The model under review builds one solid part; all positions refer to its coordinate system, in mm. A direction names the side the tool comes from. Round coordinates to 2 decimals unless told otherwise and drop trailing zeros. Write each loop counter-clockwise with the first axis right and the second up, starting at its lowest first coordinate (ties: lowest second). Pieces come first, ordered by that corner, then holes. Notation, with made-up numbers: (22.5, -7) -> (76.5, -7) arc R19 ccw to (76.5, 3) -> close; hole circle Ø5 at (34.5, 16.25). An arc over 180 degrees is marked (long way). Use CSV: the item, a comma, the result in double quotes. Start each with the question number.
1) Machinability: for faces 4 (the face through (-77, 7, -30)), 5 (the face through (-77, 15, -9.2)), 6 (the face through (-77, 20.8, -15)), 7 (the face through (-77, 15, -20.8)), which of the approach directions +Z, -Z, +X, -X, +Y, -Y give a long, thin tool a straight path to every point of the face, cutting with its end or side? Answer none if there is none.
2) Take a section at A-A, the plane z = -15. Give the boundary of the cut face in (x, y).
3) Mouldability with a two-part tool opening along Z and no side actions: class faces 1 (the face through (-77, 0, -7)), 2 (the face through (-77, 9.2, -15)), 3 (the face through (-77, 23, 0)) as released by +Z, released by -Z, zero draft, split by the parting line, or undercut.
4) Take a section at B-B, the plane y = 15. Give the boundary of the cut face in (x, z).
5) For pin 1 Ø6 at (y, z) = (25.5, -12) entering from +X; pin 2 Ø1.9 at (x, z) = (-127, -29) entering from -Y; pin 3 Ø3.5 at (x, y) = (0.5, 15) entering from +Z; pin 4 Ø1 at (x, y) = (-47, 14) entering from -Z, all flat-tipped, find the tip position at first contact; note any pin that passes through.
6) Wall thickness on probe 1 along Z at (x, y) = (9.5, 25); probe 2 along Z at (x, y) = (-36, 15); probe 3 along Y at (x, z) = (-83.5, -8): over which ranges is each line inside the solid? List them lowest first. Write a range as [from, to].
from build123d import *
from build123d.topology import SkipClean

# Parameters (mm, degrees)
SKETCH1_R           = 3.4
BOSS_EXTRUDE2_DEPTH = 100
FILLET5_R           = 2.5
FILLET6_R           = 1.5
FILLET7_R           = 1.5
FILLET8_R           = 1
SKETCH3_R           = 3.4
BOSS_EXTRUDE3_DEPTH = 140
SKETCH7_R           = 3.4
BOSS_EXTRUDE4_DEPTH = 120


with BuildPart() as part:
    # Sketch1 → Boss-Extrude2 (new body)
    with BuildSketch(Plane(origin=(0, 0, 0), x_dir=(0, 0, -1), z_dir=(1, 0, 0))):
        Polygon((10.9, 0), (10.9, 2.4), (6.75, 2.4), (6.75, 5.05), (10.9, 9.2), (19.1, 9.2), (23.25, 5.05), (23.25, 2.4), (19.1, 2.4), (19.1, 0), (30, 0), (30, 10.9), (27.6, 10.9), (27.6, 6.75), (24.95, 6.75), (20.8, 10.9), (20.8, 19.1), (24.95, 23.25), (27.6, 23.25), (27.6, 19.1), (30, 19.1), (30, 30), (19.1, 30), (19.1, 27.6), (23.25, 27.6), (23.25, 24.95), (19.1, 20.8), (10.9, 20.8), (6.75, 24.95), (6.75, 27.6), (10.9, 27.6), (10.9, 30), (0, 30), (0, 19.1), (2.4, 19.1), (2.4, 23.25), (5.05, 23.25), (9.2, 19.1), (9.2, 10.9), (5.05, 6.75), (2.4, 6.75), (2.4, 10.9), (0, 10.9), (0, 0), align=None)
        with Locations((15, 15)):
            Circle(SKETCH1_R, mode=Mode.SUBTRACT)
    extrude(amount=BOSS_EXTRUDE2_DEPTH)

    # Fillet5
    fillet5_edges = [part.edges().sort_by_distance(p)[0] for p in [
        (50, 30, 0),
        (50, 30, -30),
        (50, 0, -30),
        (50, 0, 0),
    ]]
    fillet(fillet5_edges, radius=FILLET5_R)

    # Fillet6
    fillet6_edges = [part.edges().sort_by_distance(p)[0] for p in [
        (50, 10.9, -9.2),
        (50, 19.1, -9.2),
        (50, 19.1, -20.8),
        (50, 10.9, -20.8),
        (50, 9.2, -19.1),
        (50, 9.2, -10.9),
    ]]
    fillet(fillet6_edges, radius=FILLET6_R)

    # Fillet7
    fillet7_edges = [part.edges().sort_by_distance(p)[0] for p in [
        (50, 20.8, -10.9),
        (50, 20.8, -19.1),
    ]]
    fillet(fillet7_edges, radius=FILLET7_R)

    # Fillet8
    fillet8_edges = [part.edges().sort_by_distance(p)[0] for p in [
        (50, 6.75, -2.4),
        (50, 23.25, -2.4),
        (50, 27.6, -6.75),
        (50, 27.6, -23.25),
        (50, 23.25, -27.6),
        (50, 6.75, -27.6),
        (50, 2.4, -23.25),
        (50, 2.4, -6.75),
    ]]
    fillet(fillet8_edges, radius=FILLET8_R)

    # Sketch3 → Boss-Extrude3 (add)
    with BuildSketch(Plane(origin=(0, 0, 0), x_dir=(0, 0, -1), z_dir=(1, 0, 0))):
        with BuildLine():
            Line((10.9, 27.6), (10.9, 30))
            Line((10.9, 30), (2.5, 30))
            ThreePointArc((2.5, 30), (0.732233047, 29.267766953), (0, 27.5))
            Line((0, 27.5), (0, 19.1))
            Line((0, 19.1), (2.4, 19.1))
            Line((2.4, 19.1), (2.4, 22.25))
            ThreePointArc((2.4, 22.25), (2.692893219, 22.957106781), (3.4, 23.25))
            Line((3.4, 23.25), (5.05, 23.25))
            Line((5.05, 23.25), (8.760660172, 19.539339828))
            ThreePointArc((8.760660172, 19.539339828), (9.085819299, 19.052704805), (9.2, 18.478679656))
            Line((9.2, 18.478679656), (9.2, 11.521320344))
            ThreePointArc((9.2, 11.521320344), (9.085819299, 10.947295195), (8.760660172, 10.460660172))
            Line((8.760660172, 10.460660172), (5.05, 6.75))
            Line((5.05, 6.75), (3.4, 6.75))
            ThreePointArc((3.4, 6.75), (2.692893219, 7.042893219), (2.4, 7.75))
            Line((2.4, 7.75), (2.4, 10.9))
            Line((2.4, 10.9), (0, 10.9))
            Line((0, 10.9), (0, 2.5))
            ThreePointArc((0, 2.5), (0.732233047, 0.732233047), (2.5, 0))
            Line((2.5, 0), (10.9, 0))
            Line((10.9, 0), (10.9, 2.4))
            Line((10.9, 2.4), (7.75, 2.4))
            ThreePointArc((7.75, 2.4), (7.042893219, 2.692893219), (6.75, 3.4))
            Line((6.75, 3.4), (6.75, 5.05))
            Line((6.75, 5.05), (10.460660172, 8.760660172))
            ThreePointArc((10.460660172, 8.760660172), (10.947295195, 9.085819299), (11.521320344, 9.2))
            Line((11.521320344, 9.2), (18.478679656, 9.2))
            ThreePointArc((18.478679656, 9.2), (19.052704805, 9.085819299), (19.539339828, 8.760660172))
            Line((19.539339828, 8.760660172), (23.25, 5.05))
            Line((23.25, 5.05), (23.25, 3.4))
            ThreePointArc((23.25, 3.4), (22.957106781, 2.692893219), (22.25, 2.4))
            Line((22.25, 2.4), (19.1, 2.4))
            Line((19.1, 2.4), (19.1, 0))
            Line((19.1, 0), (27.5, 0))
            ThreePointArc((27.5, 0), (29.267766953, 0.732233047), (30, 2.5))
            Line((30, 2.5), (30, 10.9))
            Line((30, 10.9), (27.6, 10.9))
            Line((27.6, 10.9), (27.6, 7.75))
            ThreePointArc((27.6, 7.75), (27.307106781, 7.042893219), (26.6, 6.75))
            Line((26.6, 6.75), (24.95, 6.75))
            Line((24.95, 6.75), (21.239339828, 10.460660172))
            ThreePointArc((21.239339828, 10.460660172), (20.914180701, 10.947295195), (20.8, 11.521320344))
            Line((20.8, 11.521320344), (20.8, 18.478679656))
            ThreePointArc((20.8, 18.478679656), (20.914180701, 19.052704805), (21.239339828, 19.539339828))
            Line((21.239339828, 19.539339828), (24.95, 23.25))
            Line((24.95, 23.25), (26.6, 23.25))
            ThreePointArc((26.6, 23.25), (27.307106781, 22.957106781), (27.6, 22.25))
            Line((27.6, 22.25), (27.6, 19.1))
            Line((27.6, 19.1), (30, 19.1))
            Line((30, 19.1), (30, 27.5))
            ThreePointArc((30, 27.5), (29.267766953, 29.267766953), (27.5, 30))
            Line((27.5, 30), (19.1, 30))
            Line((19.1, 30), (19.1, 27.6))
            Line((19.1, 27.6), (22.25, 27.6))
            ThreePointArc((22.25, 27.6), (22.957106781, 27.307106781), (23.25, 26.6))
            Line((23.25, 26.6), (23.25, 24.95))
            Line((23.25, 24.95), (19.539339828, 21.239339828))
            ThreePointArc((19.539339828, 21.239339828), (19.052704805, 20.914180701), (18.478679656, 20.8))
            Line((18.478679656, 20.8), (11.521320344, 20.8))
            ThreePointArc((11.521320344, 20.8), (10.947295195, 20.914180701), (10.460660172, 21.239339828))
            Line((10.460660172, 21.239339828), (6.75, 24.95))
            Line((6.75, 24.95), (6.75, 26.6))
            ThreePointArc((6.75, 26.6), (7.042893219, 27.307106781), (7.75, 27.6))
            Line((7.75, 27.6), (10.9, 27.6))
        make_face()
        with Locations((15, 15)):
            Circle(SKETCH3_R, mode=Mode.SUBTRACT)
    extrude(amount=-BOSS_EXTRUDE3_DEPTH)

    # Sketch7 → Boss-Extrude4 (add)
    with SkipClean():  # the faces are left unmerged after this step: merging them gives an invalid solid
        with BuildSketch(Plane.ZY.offset(140)):
            with BuildLine():
                Line((-2.4, 10.9), (0, 10.9))
                Line((0, 10.9), (0, 2.5))
                ThreePointArc((0, 2.5), (-0.732233047, 0.732233047), (-2.5, 0))
                Line((-2.5, 0), (-10.9, 0))
                Line((-10.9, 0), (-10.9, 2.4))
                Line((-10.9, 2.4), (-7.75, 2.4))
                ThreePointArc((-7.75, 2.4), (-7.042893219, 2.692893219), (-6.75, 3.4))
                Line((-6.75, 3.4), (-6.75, 5.05))
                Line((-6.75, 5.05), (-10.460660172, 8.760660172))
                ThreePointArc((-10.460660172, 8.760660172), (-10.947295195, 9.085819299), (-11.521320344, 9.2))
                Line((-11.521320344, 9.2), (-18.478679656, 9.2))
                ThreePointArc((-18.478679656, 9.2), (-19.052704805, 9.085819299), (-19.539339828, 8.760660172))
                Line((-19.539339828, 8.760660172), (-23.25, 5.05))
                Line((-23.25, 5.05), (-23.25, 3.4))
                ThreePointArc((-23.25, 3.4), (-22.957106781, 2.692893219), (-22.25, 2.4))
                Line((-22.25, 2.4), (-19.1, 2.4))
                Line((-19.1, 2.4), (-19.1, 0))
                Line((-19.1, 0), (-27.5, 0))
                ThreePointArc((-27.5, 0), (-29.267766953, 0.732233047), (-30, 2.5))
                Line((-30, 2.5), (-30, 10.9))
                Line((-30, 10.9), (-27.6, 10.9))
                Line((-27.6, 10.9), (-27.6, 7.75))
                ThreePointArc((-27.6, 7.75), (-27.307106781, 7.042893219), (-26.6, 6.75))
                Line((-26.6, 6.75), (-24.95, 6.75))
                Line((-24.95, 6.75), (-21.239339828, 10.460660172))
                ThreePointArc((-21.239339828, 10.460660172), (-20.914180701, 10.947295195), (-20.8, 11.521320344))
                Line((-20.8, 11.521320344), (-20.8, 18.478679656))
                ThreePointArc((-20.8, 18.478679656), (-20.914180701, 19.052704805), (-21.239339828, 19.539339828))
                Line((-21.239339828, 19.539339828), (-24.95, 23.25))
                Line((-24.95, 23.25), (-26.6, 23.25))
                ThreePointArc((-26.6, 23.25), (-27.307106781, 22.957106781), (-27.6, 22.25))
                Line((-27.6, 22.25), (-27.6, 19.1))
                Line((-27.6, 19.1), (-30, 19.1))
                Line((-30, 19.1), (-30, 27.5))
                ThreePointArc((-30, 27.5), (-29.267766953, 29.267766953), (-27.5, 30))
                Line((-27.5, 30), (-19.1, 30))
                Line((-19.1, 30), (-19.1, 27.6))
                Line((-19.1, 27.6), (-22.25, 27.6))
                ThreePointArc((-22.25, 27.6), (-22.957106781, 27.307106781), (-23.25, 26.6))
                Line((-23.25, 26.6), (-23.25, 24.95))
                Line((-23.25, 24.95), (-19.539339828, 21.239339828))
                ThreePointArc((-19.539339828, 21.239339828), (-19.052704805, 20.914180701), (-18.478679656, 20.8))
                Line((-18.478679656, 20.8), (-11.521320344, 20.8))
                ThreePointArc((-11.521320344, 20.8), (-10.947295195, 20.914180701), (-10.460660172, 21.239339828))
                Line((-10.460660172, 21.239339828), (-6.75, 24.95))
                Line((-6.75, 24.95), (-6.75, 26.6))
                ThreePointArc((-6.75, 26.6), (-7.042893219, 27.307106781), (-7.75, 27.6))
                Line((-7.75, 27.6), (-10.9, 27.6))
                Line((-10.9, 27.6), (-10.9, 30))
                Line((-10.9, 30), (-2.5, 30))
                ThreePointArc((-2.5, 30), (-0.732233047, 29.267766953), (0, 27.5))
                Line((0, 27.5), (0, 19.1))
                Line((0, 19.1), (-2.4, 19.1))
                Line((-2.4, 19.1), (-2.4, 22.25))
                ThreePointArc((-2.4, 22.25), (-2.692893219, 22.957106781), (-3.4, 23.25))
                Line((-3.4, 23.25), (-5.05, 23.25))
                Line((-5.05, 23.25), (-8.760660172, 19.539339828))
                ThreePointArc((-8.760660172, 19.539339828), (-9.085819299, 19.052704805), (-9.2, 18.478679656))
                Line((-9.2, 18.478679656), (-9.2, 11.521320344))
                ThreePointArc((-9.2, 11.521320344), (-9.085819299, 10.947295195), (-8.760660172, 10.460660172))
                Line((-8.760660172, 10.460660172), (-5.05, 6.75))
                Line((-5.05, 6.75), (-3.4, 6.75))
                ThreePointArc((-3.4, 6.75), (-2.692893219, 7.042893219), (-2.4, 7.75))
                Line((-2.4, 7.75), (-2.4, 10.9))
            make_face()
            with Locations((-15, 15)):
                Circle(SKETCH7_R, mode=Mode.SUBTRACT)
        extrude(amount=BOSS_EXTRUDE4_DEPTH)
    add(part.part.scale(1), mode=Mode.REPLACE)  # the faces are merged on a copy


solid = part.part
Values found:
1,face 4,"-Z, +X, -X, +Y, -Y"
1,face 5,"+Z, +X, -X"
1,face 6,"+X, -X, +Y"
1,face 7,"-Z, +X, -X"
2,outline,"(-260, 9.2) -> (100, 9.2) -> (100, 11.6) -> (-260, 11.6) -> close; (-260, 18.4) -> (100, 18.4) -> (100, 20.8) -> (-260, 20.8) -> close"
3,face 1,"zero draft"
3,face 2,"undercut"
3,face 3,"released by +Z"
4,outline,"(-260, -20.8) -> (100, -20.8) -> (100, -18.4) -> (-260, -18.4) -> close; (-260, -11.6) -> (100, -11.6) -> (100, -9.2) -> (-260, -9.2) -> close"
5,pin 1,"x = 100"
5,pin 2,"y = 0.06"
5,pin 3,"z = -9.2"
5,pin 4,"z = -20.8"
6,probe 1,"[-30, -23.25], [-6.75, 0]"
6,probe 2,"[-20.8, -18.4], [-11.6, -9.2]"
6,probe 3,"[0, 2.4], [6.3, 9.7], [20.3, 23.7], [27.6, 30]"
